Check sheet for the modelled part. Datum: model origin and axes. Units: mm. Face numbers are marked on the shaded views. A direction names the side the tool comes from. Give positions to 0.01 mm unless a question says otherwise; leave off trailing zeros. Write each loop counter-clockwise with the first axis right and the second up, starting at its lowest first coordinate (ties: lowest second). Pieces come first, ordered by that corner, then holes. Notation, with made-up numbers: (82.25, -1) -> (122.25, -1) arc R27 ccw to (122.25, 16) -> close; hole circle Ø7 at (-18, 40). An arc over 180 degrees is marked (long way). Return JSON: item names as keys, results as strings.
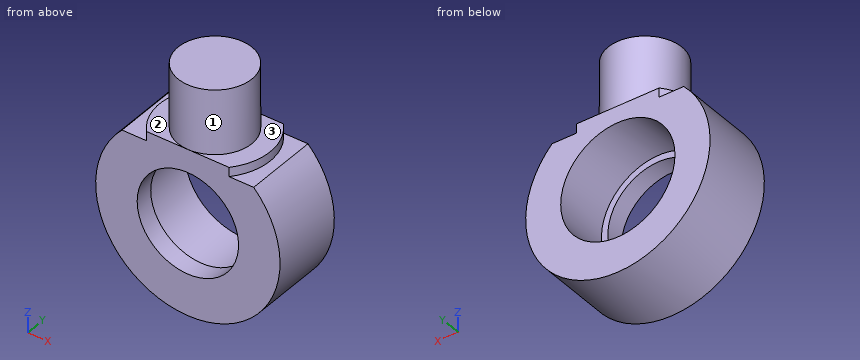
Autodesk Inventor part; units mm, degrees
ref_plane "YZ Plane" through (0, 0, 0) normal (1, 0, 0) x (0, 1, 0)
ref_plane "XZ Plane" through (0, 0, 0) normal (0, 1, 0) x (-1, 0, 0)
ref_plane "XY Plane" through (0, 0, 0) normal (0, 0, 1) x (1, 0, 0)
sketch "Sketch1" plane through (0, 0, 0) normal (0, 1, 0) x (-1, 0, 0)
  line L0 (0, -19.6) -> (0, 19.6)
  line L1 (19.6, 0) -> (-19.6, 0)
  circle A0 centre (0, 0) radius 2
  circle A1 centre (0, 0) radius 6.2
  circle A2 centre (0, 0) radius 14
  line L2 (4, -13.4164) -> (-4, -13.4164)
  circle A3 centre (0, 0) radius 10
  line L3 (6, 8) -> (-6, 8)
  line L4 (7.1414, 7) -> (-7.1414, 7)
  dimension "d0" = 4
  dimension "d1" = 12.4
  dimension "d2" = 28
  dimension "d3" = 8
  dimension "d4" = 20
  dimension "d5" = 12
  dimension "d7" = 1
extrude "Extrusion1" add sketch "Sketch1" along normal blind 8 contours A3 L1 A1 L0 | L0 A1 L1 A3 | A3 L4 L0 A1 L1 | L1 A1 L0 L4 A3
sketch "Sketch2" plane through (-7.1414, 0, 7) normal (0, 0, 1) x (1, 0, 0)
  line L0 (0, 0) -> (14.2829, 0)
  line L1 (14.2829, 0) -> (14.2829, 8)
  line L2 (0, 8) -> (14.2829, 8)
  line L3 (0, 0) -> (0, 8)
  line L4 (7.1414, -4) -> (7.1414, 10)
  line L5 (2.6693, 8) -> (11.6136, 8)
  line L6 (2.6693, 0) -> (11.6136, 0)
  arc A0 (2.6693, 8) -> (2.6693, 0) centre (7.1414, 4) ccw
  arc A1 (11.6136, 0) -> (11.6136, 8) centre (7.1414, 4) ccw
  point P0 (7.1414, 0)
  dimension "d10" = 4
  dimension "d26" = 8
  dimension "d27" = 6
  dimension "d28" = 6
extrude "Extrusion2" add sketch "Sketch2" along normal blind 1 contours A0 L2 L4 L0 | L4 L2 A1 L0
sketch "Sketch3" plane through (-7.1414, 0, 8) normal (0, 0, 1) x (1, 0, 0)
  arc A0 (2.6693, 8) -> (2.6693, 0) centre (7.1414, 4) ccw
  circle A1 centre (7.1414, 4) radius 4
  point P0 (7.1414, 0)
  point P1 (6.5905, 0)
  point P2 (6.5905, 4)
  dimension "d14" = 8
extrude "Extrusion3" add sketch "Sketch3" along normal blind 7
sketch "Sketch4" plane through (0, 0, 0) normal (0, 1, 0) x (-1, 0, 0)
  circle A0 centre (0, 0) radius 5.5
  circle A1 centre (0, 0) radius 6.2
  circle A2 centre (0, 0) radius 6.5
  dimension "d29" = 11
  dimension "d30" = 13
extrude "Extrusion4" add sketch "Sketch4" along normal blind 2 contours A1
properties part number "borde libre chico"
(1) Set-up check for the marked faces 1, 2 and 3: record each of +Z, -Z, +X, -X, +Y, -Y from which the full face is reachable in a straight line by a thin tool's end or side.
Reply:
{"face 1": "+Z", "face 2": "+Z, -X", "face 3": "+Z, +X"}
(2) Cross-section at B-B on y = 6.5. Enter the section's corners in (x, z), then the cut area to 3 significant figures.
Reply:
{"outline": "(-7.14, 7) arc R10 ccw (long way) to (7.14, 7) -> (5.45, 7) -> (5.45, 8) -> (3.12, 8) -> (3.12, 15) -> (-3.12, 15) -> (-3.12, 8) -> (-5.45, 8) -> (-5.45, 7) -> close; hole circle Ø12.4 at (0, 0)", "area": "218 mm^2"}
(3) Cross-section at A-A on z = -1.75. Enter the section's corners in (x, y).
Reply:
{"outline": "(-9.85, 0) -> (-5.21, 0) -> (-5.21, 2) -> (-5.95, 2) -> (-5.95, 8) -> (-9.85, 8) -> close; (5.21, 0) -> (9.85, 0) -> (9.85, 8) -> (5.95, 8) -> (5.95, 2) -> (5.21, 2) -> close"}
(4) Thickness scan on L1, parallel to Z at x = 0, y = 1.2; L2, parallel to Z at x = 0, y = 3.55; L3, parallel to X at y = 6.3, z = 0. Record the ranges inside material, lowest first.
Reply:
{"L1": "-10 to -5.5, 5.5 to 15", "L2": "-10 to -6.2, 6.2 to 15", "L3": "-10 to -6.2, 6.2 to 10"}
(5) Depth check by flat-ended pin: pin 1 Ø10 at (x, z) = (0, 0) entering from -Y; pin 2 Ø10 at (x, z) = (0.5, 2) entering from +Y; pin 3 Ø1.3 at (x, y) = (6.5, 6) entering from +Z; pin 4 Ø2 at (x, y) = (-6, 4.5) entering from +Z. Enter the tip coordinate at first touch or a pass-through.
Reply:
{"pin 1": "through", "pin 2": "y = 8", "pin 3": "z = 7", "pin 4": "z = 8"}
(6) Cross-section at D-D on z = 12.5. Enter the section's corners in (x, y).
Reply:
{"outline": "circle Ø8 at (0, 4)"}
(7) Cross-section at C-C on x = -0.75. Enter the section's corners in (y, z).
Reply:
{"outline": "(0, -9.97) -> (8, -9.97) -> (8, -6.15) -> (2, -6.15) -> (2, -5.45) -> (0, -5.45) -> close; (0, 5.45) -> (2, 5.45) -> (2, 6.15) -> (8, 6.15) -> (8, 8) -> (7.93, 8) -> (7.93, 15) -> (0.07, 15) -> (0.07, 8) -> (0, 8) -> close"}
